Geometry check sheet. Reference: the model listing, model coordinates, mm. Give positions to 0.01 mm unless a question says otherwise; leave off trailing zeros. Write each loop counter-clockwise with the first axis right and the second up, starting at its lowest first coordinate (ties: lowest second). Pieces come first, ordered by that corner, then holes. Notation, with made-up numbers: (43, -33) -> (91, -33) arc R11 cw to (91, -28) -> close; hole circle Ø3 at (11.25, 41). An arc over 180 degrees is marked (long way). Write item = value, one per line. Start each with the question number.
1. Cross-section at A-A, the plane y = -5.76. Record the cut outline in (x, z), plus the area to 3 significant figures.
2. Depth check by flat-ended pin: P1, Ø5, axis at y = -5.76, z = 25, coming from the +X side; P2, Ø2.5, axis at y = -5.76, z = 5, coming from the +X side; P3, Ø3, axis at x = -93, z = 19, coming from the -Y side. Enter the tip coordinate at first touch or a pass-through.
3. Thickness scan on line 1 along Z through (x, y) = (-300.2, -5.76); line 2 along Y through (x, z) = (300.2, 25); line 3 along X through (y, z) = (-5, 7). Record the ranges inside material, lowest first.
4. Cross-section at B-B, the plane x = -256. Record the cut outline in (y, z).
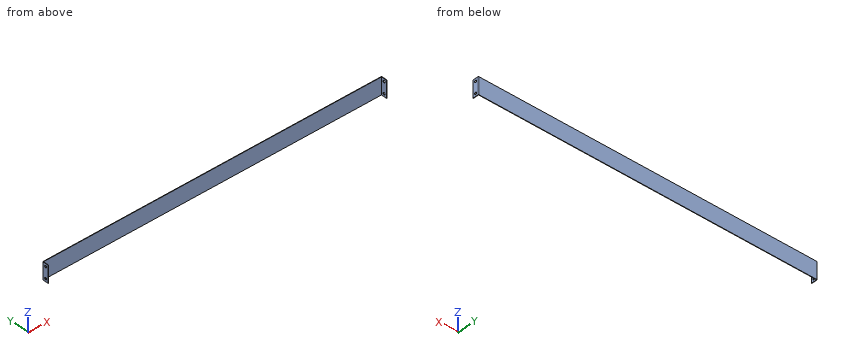
Autodesk Inventor part; units mm, degrees
ref_plane "Work Plane1" through (300.76, -10.76, 30) normal (1, 0, 0) x (0, 0, -1)
ref_plane "Work Plane2" through (-300.76, -10.76, 0) normal (-1, 0, 0) x (0, 0, 1)
ref_plane "YZ Plane" through (0, 0, 0) normal (1, 0, 0) x (0, 1, 0)
sketch "Sketch1" plane through (0, 0, 0) normal (0, 0, 1) x (1, 0, 0)
  line L0 (-300, 0) -> (300, 0)
  line L1 (-300, -0.76) -> (300, -0.76)
  line L2 (-300, -0.76) -> (-300, -10.76)
  line L3 (-300, -10.76) -> (-300.76, -10.76)
  line L4 (-300.76, -10.76) -> (-300.76, 0)
  line L5 (-300.76, 0) -> (-300, 0)
  line L6 (300, -0.76) -> (300, -10.76)
  line L7 (300, -10.76) -> (300.76, -10.76)
  line L8 (300.76, -10.76) -> (300.76, 0)
  line L9 (300.76, 0) -> (300, 0)
  point P0 (0, 0)
  point P1 (0, 0)
  dimension "d0" = 600
  dimension "d2" = 0.76
  dimension "d3" = 10
  dimension "d4" = 0.76
  dimension "d5" = 300
  dimension "d6" = 600
  dimension "d7" = 10
  dimension "d8" = 0.76
extrude "Extrusion1" add sketch "Sketch1" along normal blind 30
fillet "Fillet1" radius 1 1 edges at (-300.76, 0, 15)
fillet "Fillet2" radius 1 1 edges at (300.76, 0, 15)
ref_plane "Work Plane1" through (300.76, -10.76, 30) normal (1, 0, 0) x (0, 0, -1)
sketch "Sketch2" plane through (300.76, -10.76, 30) normal (1, 0, 0) x (0, 0, -1)
  line L0 (0, 9.76) -> (30, 9.76)
  line L1 (0, 0) -> (0, 9.76)
  line L2 (30, 0) -> (0, 0)
  line L3 (30, 9.76) -> (30, 0)
  point P0 (30, 10.76)
  point P1 (5, 5)
  point P2 (25, 5)
  dimension "d14" = 5
  dimension "d15" = 5
  dimension "d16" = 5
  dimension "d17" = 5
hole "Hole1" at (300.76, -5.76, 25) at (300.76, -5.76, 5) direction (-1, 0, 0) diameter 4 depth 0.76 tip angle 118
ref_plane "Work Plane2" through (-300.76, -10.76, 0) normal (-1, 0, 0) x (0, 0, 1)
sketch "Sketch3" plane through (-300.76, -10.76, 0) normal (-1, 0, 0) x (0, 0, 1)
  line L0 (0, 0) -> (30, 0)
  line L1 (0, 0) -> (0, 9.76)
  line L2 (30, 9.76) -> (30, 0)
  point P0 (0, 10.76)
  point P1 (5, 5)
  point P2 (25, 5)
  dimension "d26" = 5
  dimension "d27" = 5
  dimension "d28" = 5
  dimension "d29" = 5
hole "Hole2" at (-300.76, -5.76, 5) at (-300.76, -5.76, 25) direction (1, 0, 0) diameter 4 depth 0.76 tip angle 118
equation "\"BendRadius\" = Thickness"
equation "\"BendReliefWidth\" = Thickness"
equation "\"BendReliefDepth\" = 0.5 * Thickness"
equation "\"CornerReliefSize\" = 4 * Thickness"
equation "\"MinimumRemnant\" = 2 * Thickness"
equation "\"TransitionRadius\" = BendRadius"
equation "\"JacobiRadiusSize\" = BendRadius"
equation "\"GapSize\" = Thickness"
properties part number "Fin" material "Stainless Steel"
Answers:
q1.outline = (-300.76, 0) -> (-300, 0) -> (-300, 3) -> (-300.76, 3) -> close; (-300.76, 7) -> (-300, 7) -> (-300, 23) -> (-300.76, 23) -> close; (-300.76, 27) -> (-300, 27) -> (-300, 30) -> (-300.76, 30) -> close; (300, 0) -> (300.76, 0) -> (300.76, 3) -> (300, 3) -> close; (300, 7) -> (300.76, 7) -> (300.76, 23) -> (300, 23) -> close; (300, 27) -> (300.76, 27) -> (300.76, 30) -> (300, 30) -> close
q1.area = 33.4 mm^2
q2.P1 = 300.76
q2.P2 = through
q2.P3 = -0.76
q3.line_1 = 0 to 3, 7 to 23, 27 to 30
q3.line_2 = -10.76 to -7.76, -3.76 to -0.1
q3.line_3 = -300.76 to -300, 300 to 300.76
q4.outline = (-0.76, 0) -> (0, 0) -> (0, 30) -> (-0.76, 30) -> close
